Geometry: see drawing. Coordinates: mm, zero at the bounding-box minimum. Round coordinates to 2 decimals unless told otherwise and drop trailing zeros. Order: outer loops, then holes, each group sorted by start corner. A loop starts at its lowest first (then second) coordinate and runs counter-clockwise, first axis right, second up. Notation, with made-up numbers: (54, 24.25) -> (79, 24.25) arc R20 ccw to (79, 62.25) -> close; hole circle Ø8 at (-31, 38). An arc over 180 degrees is marked (long way). Use a Markdown table: item, result.
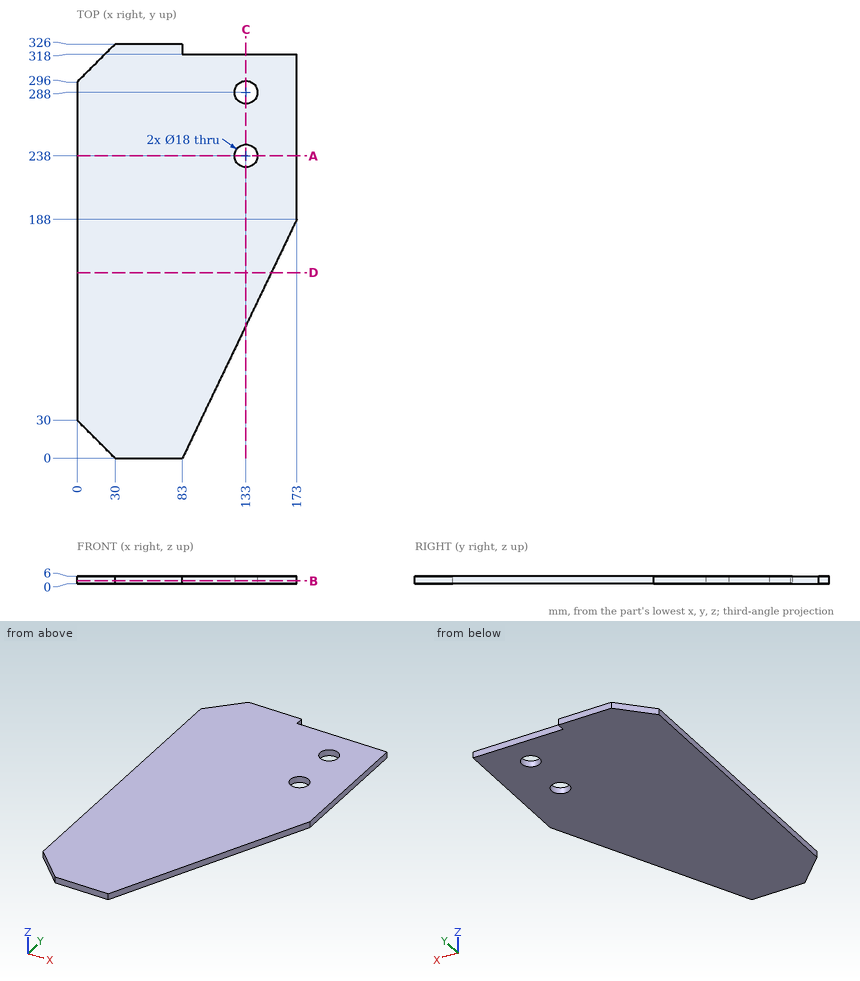
1) Cut plane B-B on z = 2.3. Return loops of the section in (x, y).
Answer key:
| item | result |
|---|---|
| outline | (0, 30) -> (30, 0) -> (83, 0) -> (173, 188) -> (173, 318) -> (83, 318) -> (83, 326) -> (30, 326) -> (0, 296) -> close; hole circle Ø18 at (133, 238); hole circle Ø18 at (133, 288) |
2) Contact query for flat-ended pins moving along their axis: P1, Ø3, axis at y = 88.5, z = 1, coming from the +X side; P2, Ø3, axis at y = 154.5, z = 1, coming from the +X side. Output: stop coordinate, or through.
Answer key:
| item | result |
|---|---|
| P1 | stops at x = 126.09 |
| P2 | stops at x = 157.68 |
3) Cut plane D-D on y = 146. Return loops of the section in (x, z).
Answer key:
| item | result |
|---|---|
| outline | (0, 0) -> (152.89, 0) -> (152.89, 6) -> (0, 6) -> close |
4) Ray query, probe 1 along X at (y, z) = (238, 1.75); probe 2 along Y at (x, z) = (127.5, 2.4); probe 3 along Y at (x, z) = (133, 2.9). Return the intervals inside material, ascending.
Answer key:
| item | result |
|---|---|
| probe 1 | x = 0 to 124, 142 to 173 |
| probe 2 | y = 92.96 to 230.88, 245.12 to 280.88, 295.12 to 318 |
| probe 3 | y = 104.44 to 229, 247 to 279, 297 to 318 |
5) Cut plane A-A on y = 238. Return loops of the section in (x, z), and give its area (3 significant figures).
Answer key:
| item | result |
|---|---|
| outline | (0, 0) -> (124, 0) -> (124, 6) -> (0, 6) -> close; (142, 0) -> (173, 0) -> (173, 6) -> (142, 6) -> close |
| area | 930 mm^2 |
6) Cut plane C-C on x = 133. Return loops of the section in (y, z).
Answer key:
| item | result |
|---|---|
| outline | (104.44, 0) -> (229, 0) -> (229, 6) -> (104.44, 6) -> close; (247, 0) -> (279, 0) -> (279, 6) -> (247, 6) -> close; (297, 0) -> (318, 0) -> (318, 6) -> (297, 6) -> close |
